from build123d import *

# Parameters (mm, degrees)
F0_R     = 13.9349821394
F1_DEPTH = 20
F3_D     = 3.3
F3_DEPTH = 5
F3_TIP   = 0.9914200214


with BuildPart() as f1:
    # F0 (on Right) → F1 (new body)
    with BuildSketch(Plane.YZ):
        Polygon((-65.3123139198, 200), (-65.3123139198, 100), (34.6876860802, 100), align=None)
        Polygon((-65.3123139198, 100), (-65.3123139198, 0), (-45.3123139198, 0), (-45.3123139198, 19.40359734), (-25.3123139198, 19.40359734), (-25.3123139198, 0), (-5.3123139198, 0), (-5.3123139198, 20), (14.6876860802, 20), (14.6876860802, 0), (34.6876860802, 0), (34.6876860802, 100), align=None)
        with Locations((-35.3123139198, 70)):
            Circle(F0_R, mode=Mode.SUBTRACT)
    extrude(amount=F1_DEPTH)

    # F3
    with Locations(Plane(origin=(0, 67.3438430401, 67.3438430401), x_dir=(-1, 0, 0), z_dir=(0, 0.7071067812, 0.7071067812))):
        with Locations((-10, 56.1827800676), (-10, 156.1827800676)):
            Hole(F3_D / 2, depth=F3_DEPTH)
            with Locations((0, 0, -(F3_DEPTH + F3_TIP / 2))):  # 118° drill point
                Cone(0, F3_D / 2, F3_TIP, mode=Mode.SUBTRACT)


solid = f1.part
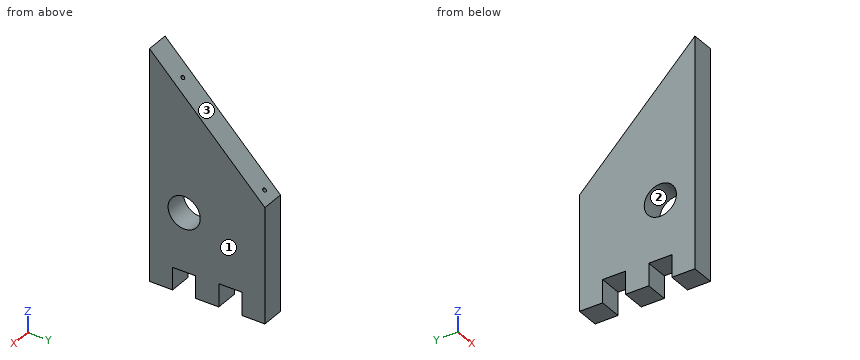
The model under review builds one solid part; all positions refer to its coordinate system, in mm. Face numbers are marked on the shaded views. Coordinates: 2 decimals unless noted, no trailing zeros. Write each loop counter-clockwise with the first axis right and the second up, starting at its lowest first coordinate (ties: lowest second). Pieces come first, ordered by that corner, then holes. Notation, with made-up numbers: (77, 89.25) - (109, 89.25) arc R23 cw to (109, 121.25) - close; hole circle Ø1 at (2.5, 48). An arc over 180 degrees is marked (long way). Answer as a JSON object with one key per item and string values. Group by question number.
1. Add section C-C (y = -38). Give the boundary of the cut face in (x, z), plus the area to 3 significant figures.
2. To check wall thickness, follow probe 1 along Y at (x, z) = (16, 8); probe 2 along Y at (x, z) = (11.25, 78); probe 3 along Y at (x, z) = (4.5, 62.5). State the ranges of each line that lie inside material, in increasing order.
3. Add section B-B (z = 70). Give the boundary of the cut face in (x, y), plus the area to 3 significant figures.
4. Mouldability with a two-part tool opening along Y and no side actions: class the marked faces 1, 2 and 3 as pulls with the +Y half, pulls with the -Y half, needs draft (parallel to the pull), parting line crosses it, or undercut.
5. Clearance check with flat-ended pins moving along their axes: pin 1 Ø6 at (x, y) = (10, 21.5) entering from -Z; pin 2 Ø1 at (x, y) = (7.5, 23) entering from +Z; pin 3 Ø8 at (x, y) = (10, -50.5) entering from +Z. State where each tip first meets the part, or that it passes through.
6. Add section D-D (z = 184.5). Give the boundary of the cut face in (x, y), plus the area to 3 significant figures.
7. Add section A-A (x = 6). Give the boundary of the cut face in (y, z).
Findings:
{
 "1": {"outline": "(0, 19.4) - (20, 19.4) - (20, 56.33) - (0, 56.33) - close; (0, 83.67) - (20, 83.67) - (20, 172.69) - (0, 172.69) - close", "area": "2,520 mm²"},
 "2": {"probe 1": "-65.31 to -45.31, -25.31 to -5.31, 14.69 to 34.69", "probe 2": "-65.31 to -46.72, -23.9 to 34.69", "probe 3": "-65.31 to -47.06, -23.57 to 34.69"},
 "3": {"outline": "(0, -65.31) - (20, -65.31) - (20, -49.25) - (0, -49.25) - close; (0, -21.38) - (20, -21.38) - (20, 34.69) - (0, 34.69) - close", "area": "1,440 mm²"},
 "4": {"face 1": "needs draft", "face 2": "undercut", "face 3": "pulls with the +Y half"},
 "5": {"pin 1": "z = 0", "pin 2": "z = 112.19", "pin 3": "z = 189.19"},
 "6": {"outline": "(0, -65.31) - (20, -65.31) - (20, -49.81) - (0, -49.81) - close", "area": "310 mm²"},
 "7": {"outline": "(-65.31, 0) - (-45.31, 0) - (-45.31, 19.4) - (-25.31, 19.4) - (-25.31, 0) - (-5.31, 0) - (-5.31, 20) - (14.69, 20) - (14.69, 0) - (34.69, 0) - (34.69, 100) - (-65.31, 200) - close; hole circle Ø27.87 at (-35.31, 70)"}
}
